CAD build for the part. Positions are in the model's coordinates, mm. Round coordinates to 2 decimals unless told otherwise and drop trailing zeros. Loops run counter-clockwise (first coordinate to the right, second up) from the corner with the lowest first, then second, coordinate; pieces in that order, holes last.
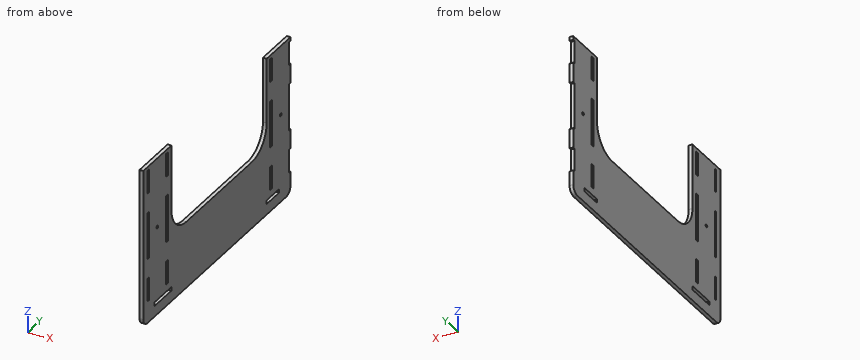
Autodesk Inventor part; units mm, degrees
ref_plane "YZ Plane" through (0, 0, 0) normal (1, 0, 0) x (0, 1, 0)
ref_plane "XZ Plane" through (0, 0, 0) normal (0, 1, 0) x (-1, 0, 0)
ref_plane "XY Plane" through (0, 0, 0) normal (0, 0, 1) x (1, 0, 0)
sketch "Sketch1" plane through (0, 0, 0) normal (1, 0, 0) x (0, 1, 0)
  line L0 (-181.2435, 115.0382) -> (-181.2435, -87.4618)
  line L1 (-80.2478, -7.4618) -> (73.7522, -7.4618)
  line L2 (-171.2435, -97.4618) -> (154.7524, -97.4618)
  line L3 (164.7524, -67.9618) -> (164.7524, -87.4618)
  circle A0 centre (141.7569, 21.2887) radius 2
  line L4 (-117.2477, 115.0382) -> (-181.2435, 115.0382)
  line L5 (-117.2477, 115.0382) -> (-115.2478, 115.0382)
  line L6 (-115.2478, 115.0382) -> (-115.2478, 27.5382)
  line L7 (108.7522, 27.5382) -> (108.7522, 115.0382)
  line L8 (108.7522, 115.0382) -> (164.7524, 115.0382)
  arc A1 (-181.2435, -87.4618) -> (-171.2435, -97.4618) centre (-171.2435, -87.4618) ccw
  line L9 (-128.2203, -67.9618) -> (-128.2203, -36.7118)
  line L10 (-128.2203, -36.7118) -> (-123.2203, -36.7118)
  line L11 (-123.2203, -67.9618) -> (-123.2203, -36.7118)
  line L12 (-128.2203, -67.9618) -> (-123.2203, -67.9618)
  line L13 (-128.2203, -10.4618) -> (-128.2203, 52.5382)
  line L14 (-128.2203, -10.4618) -> (-123.2203, -10.4618)
  line L15 (-123.2203, -10.4618) -> (-123.2203, 52.5382)
  line L16 (-128.2203, 52.5382) -> (-123.2203, 52.5382)
  line L17 (-128.2203, 78.7882) -> (-123.2203, 78.7882)
  line L18 (-123.2203, 78.7882) -> (-123.2203, 110.0382)
  line L19 (-128.2203, 110.0382) -> (-123.2203, 110.0382)
  line L20 (-128.2203, 78.7882) -> (-128.2203, 110.0382)
  circle A2 centre (-148.2261, 21.2878) radius 2
  line L21 (121.7524, 78.7882) -> (121.7524, 110.0382)
  line L22 (121.7524, 110.0382) -> (116.7524, 110.0382)
  line L23 (116.7524, 78.7882) -> (116.7524, 110.0382)
  line L24 (121.7524, 78.7882) -> (116.7524, 78.7882)
  line L25 (121.7524, -10.4618) -> (121.7524, 52.5382)
  line L26 (121.7524, 52.5382) -> (116.7524, 52.5382)
  line L27 (116.7524, -10.4618) -> (116.7524, 52.5382)
  line L28 (121.7524, -10.4618) -> (116.7524, -10.4618)
  line L29 (121.7524, -67.9618) -> (121.7524, -36.7118)
  line L30 (121.7524, -36.7118) -> (116.7524, -36.7118)
  line L31 (116.7524, -67.9618) -> (116.7524, -36.7118)
  line L32 (121.7524, -67.9618) -> (116.7524, -67.9618)
  line L33 (164.7524, 110.0382) -> (164.7524, 115.0382)
  line L34 (161.7524, 110.0382) -> (164.7524, 110.0382)
  line L35 (161.7524, 78.7882) -> (161.7524, 110.0382)
  line L36 (164.7524, 78.7882) -> (161.7524, 78.7882)
  line L37 (164.7524, 52.5382) -> (164.7524, 78.7882)
  line L38 (161.7524, 52.5382) -> (164.7524, 52.5382)
  line L39 (161.7524, -10.4618) -> (161.7524, 52.5382)
  line L40 (164.7524, -10.4618) -> (161.7524, -10.4618)
  line L41 (164.7524, -36.7118) -> (164.7524, -10.4618)
  line L42 (161.7524, -36.7118) -> (164.7524, -36.7118)
  line L43 (161.7524, -67.9618) -> (161.7524, -36.7118)
  line L44 (164.7524, -67.9618) -> (161.7524, -67.9618)
  arc A3 (73.7522, -7.4618) -> (108.7522, 27.5382) centre (73.7522, 27.5382) ccw
  arc A4 (-115.2478, 27.5382) -> (-80.2478, -7.4618) centre (-80.2478, 27.5382) ccw
  line L45 (-155.2478, -82.9618) -> (-115.2478, -82.9618)
  line L46 (-115.2478, -82.9618) -> (-115.2478, -77.9618)
  line L47 (-155.2478, -77.9618) -> (-115.2478, -77.9618)
  line L48 (-155.2478, -82.9618) -> (-155.2478, -77.9618)
  line L49 (108.7522, -82.9618) -> (138.0022, -82.9618)
  line L50 (138.0022, -82.9618) -> (138.0022, -77.9618)
  line L51 (108.7522, -77.9618) -> (138.0022, -77.9618)
  line L52 (108.7522, -82.9618) -> (108.7522, -77.9618)
  arc A5 (154.7524, -97.4618) -> (164.7524, -87.4618) centre (154.7524, -87.4618) ccw
  line L53 (-168.221, -67.9618) -> (-171.221, -67.9618)
  line L54 (-171.221, -36.7118) -> (-171.221, -67.9618)
  line L55 (-168.221, -36.7118) -> (-168.221, -67.9618)
  line L56 (-168.221, -36.7118) -> (-171.221, -36.7118)
  line L57 (-168.221, -10.4618) -> (-171.221, -10.4618)
  line L58 (-168.221, 52.5382) -> (-168.221, -10.4618)
  line L59 (-171.221, 52.5382) -> (-171.221, -10.4618)
  line L60 (-168.221, 52.5382) -> (-171.221, 52.5382)
  line L61 (-168.221, 78.7882) -> (-171.221, 78.7882)
  line L62 (-171.221, 110.0382) -> (-171.221, 78.7882)
  line L63 (-168.221, 110.0382) -> (-168.221, 78.7882)
  line L64 (-168.221, 110.0382) -> (-171.221, 110.0382)
  point P0 (141.7524, 19.2994)
  point P1 (143.3399, 20.8869)
  point P2 (164.7524, -92.4608)
  point P3 (161.7524, -97.4618)
  point P4 (-176.2435, -97.4618)
  point P5 (-181.2435, -92.4608)
  point P6 (-115.2478, 7.8284)
  point P7 (-107.2347, -7.4618)
  point P8 (98.7522, -7.4618)
  point P9 (108.7522, 9.8153)
  point P10 (156.7524, -97.4618)
  point P11 (-95.2478, -7.4618)
  point P12 (-115.2478, 12.5382)
  dimension "d40" = 212.5
  dimension "d41" = 212.5
  dimension "d44" = 4
  dimension "d50" = 35
  dimension "d51" = 90
  dimension "d52" = 35
  dimension "d54" = 3
  dimension "d55" = 10
extrude "Extrusion1" add sketch "Sketch1" along normal blind 5
properties part number "side bracer" material "Brass, Soft Yellow"
Item 1: Cut at A-A (z = -63). List the corners of the cut face in (x, y).
Verdict:
outline: (0, -181.24) - (5, -181.24) - (5, -171.22) - (0, -171.22) - close; (0, -168.22) - (5, -168.22) - (5, -128.22) - (0, -128.22) - close; (0, -123.22) - (5, -123.22) - (5, 116.75) - (0, 116.75) - close; (0, 121.75) - (5, 121.75) - (5, 161.75) - (0, 161.75) - close
Item 2: Wall check: L1, parallel to Z at x = 4.6, y = 119; L2, parallel to Y at x = 1.55, z = 32; L3, parallel to Z at x = 3.7, y = -151.5. Give the ranges that are in metal, low to high.
Verdict:
L1: z = -97.46 to -82.96, -77.96 to -67.96, -36.71 to -10.46, 52.54 to 78.79, 110.04 to 115.04
L2: y = -181.24 to -171.22, -168.22 to -128.22, -123.22 to -115.25, 108.75 to 116.75, 121.75 to 161.75
L3: z = -97.46 to -82.96, -77.96 to 115.04
Item 3: Cut at B-B (y = -134.5). List the corners of the cut face in (x, z), plus the area to 3 significant figures.
Verdict:
outline: (0, -97.46) - (5, -97.46) - (5, -82.96) - (0, -82.96) - close; (0, -77.96) - (5, -77.96) - (5, 115.04) - (0, 115.04) - close
area: 1,040 mm2
Item 4: Flat gauge pins, fed straight in: P1, Ø5, axis at y = 141.76, z = 21.29, coming from the -X side; P2, Ø12, axis at y = 99, z = 54.5, coming from the +X side; P3, Ø2.5, axis at x = 1.5, z = -47.5, coming from the +Y side. Where does each tip first touch, or does it go through?
Verdict:
P1: stops at x = 0
P2: passes through
P3: stops at y = 161.75
Item 5: Cut at C-C (z = 74). List the corners of the cut face in (x, y).
Verdict:
outline: (0, -181.24) - (5, -181.24) - (5, -115.25) - (0, -115.25) - close; (0, 108.75) - (5, 108.75) - (5, 164.75) - (0, 164.75) - close
Item 6: Cut at D-D (y = -76.5). List the corners of the cut face in (x, z).
Verdict:
outline: (0, -97.46) - (5, -97.46) - (5, -7.46) - (0, -7.46) - close
